Model file for the job. Use its own axes, mm. Face numbers are marked on the shaded views. A direction names the side the tool comes from. Round coordinates to 2 decimals unless told otherwise and drop trailing zeros. Order: outer loops, then holes, each group sorted by start corner. A loop starts at its lowest first (then second) coordinate and runs counter-clockwise, first axis right, second up. Notation, with made-up numbers: M 19.5,0 L 38.5,0 A22 ccw 38.5,21 Z; hole C 23.5,62.25 d11. An arc over 180 degrees is marked long. Return JSON: item names as keys, results as strings. Group by question number.
Item 1: Pull direction X, two halves, no side cores. Call the marked faces 1, 2 and 3: pulls with the +X half, pulls with the -X half, needs draft (parallel to the pull), parting line crosses it, or undercut.
Item 2: Pin check, flat tips, straight feed: pin 1 Ø1.5 at (x, z) = (0, 23) entering from +Y; pin 2 Ø3.5 at (x, z) = (12, 18) entering from -Y; pin 3 Ø0.9 at (x, z) = (-11.5, 16.5) entering from +Y. Stop position of each tip, or through.
Item 3: Slice it at B-B on x = -4.75. Write the cut outline in (y, z).
Item 4: Slice it at A-A on y = 19. Write the cut outline in (x, z).
Item 5: Slice it at D-D on z = 5.5. Write the cut outline in (x, y), then the cut area to 3 significant figures.
Item 6: Slice it at C-C on z = 21.25. Write the cut outline in (x, y), then the cut area to 3 significant figures.
Item 7: Probe line 1 along X through (y, z) = (13.5, 17.75); line 2 along Z through (x, y) = (-10.75, -20); line 3 along Y through (x, z) = (5.75, 10.75). List the from-to ranges inside material, lowest first.
Item 8: Which spindle directions (+Z, -Z, +X, -X, +Y, -Y) get a long thin tool onto all of the face, cutting with end or side? Do the marked faces 4, 5, 6, 7 and 8. Say none if no direction does.
Autodesk Fusion 360 part; units mm, degrees
sketch "Schizzo1" plane through (0, 0, 0) normal (0, 0, 1) x (1, 0, 0)
  line L0 (12.7, -24.75) -> (-12.7, -24.75)
  line L1 (-12.7, -24.75) -> (-12.7, 24.75)
  line L2 (12.7, 24.75) -> (12.7, -24.75)
  line L3 (12.7, -24.75) -> (-12.7, 24.75) construction
  line L4 (-12.7, -24.75) -> (12.7, 24.75) construction
  line L5 (9.7, -18.25) -> (-9.7, -18.25)
  line L6 (9.7, 21.75) -> (9.7, -18.25)
  line L7 (-9.7, -18.25) -> (-9.7, 21.75)
  line L8 (-12.7, 24.75) -> (-9.7, 24.75)
  line L9 (9.7, 24.75) -> (12.7, 24.75)
  line L10 (-9.7, 21.75) -> (-6.7, 21.75)
  line L11 (-6.7, 21.75) -> (-9.7, 24.75)
  line L12 (9.7, 21.75) -> (6.7, 21.75)
  line L13 (6.7, 21.75) -> (9.7, 24.75)
  line L14 (-9.7, -18.25) -> (-12.7, -18.25)
  line L15 (9.7, -18.25) -> (12.7, -18.25)
  line L16 (-9.7, 21.75) -> (-12.7, 21.75)
  line L17 (9.7, 21.75) -> (12.7, 21.75)
  dimension "d15" = 19.4
  dimension "d16" = 3
  dimension "d17" = 3
  dimension "d18" = 6.5
  dimension "d19" = 43
  dimension "d20" = 3
  dimension "d22" = 3
  dimension "d23" = 3
  dimension "d24" = 3
extrude "Estrusione2" add sketch "Schizzo1" along normal blind 25 contours L0 L1 L2 L5 L14 L15 | L2 L6 L15 L17 | L1 L7 L14 L16
extrude "Estrusione3" add sketch "Schizzo1" along normal blind 15 contours L2 L9 L12 L13 L17 | L1 L8 L10 L11 L16
extrude "Estrusione4" cut sketch "Schizzo1" along normal blind 5 from surface at 15 contours L0 L1 L2 L5 L14 L15
chamfer "Smusso1" distance 5 angle 45 2 edges at (11.2, 21.75, 25) (-11.2, 21.75, 25)
sketch "Schizzo2" plane through (0, -24.75, 0) normal (0, -1, 0) x (1, 0, 0)
  line L0 (12.7, 15) -> (-12.7, 15)
  line L1 (-12.7, 15) -> (-12.7, 0)
  line L2 (-12.7, 0) -> (12.7, 0)
  line L3 (12.7, 0) -> (12.7, 15)
  line L4 (0, 15) -> (0, 0) construction
  circle A0 centre (0, 9.5) radius 2.5
  line L5 (-2, 11) -> (2, 11)
  line L6 (-2, 8) -> (2, 8)
  line L7 (-2.5, 9.5) -> (2.5, 9.5) construction
  dimension "d33" = 5
  dimension "d34" = 3
  dimension "d35" = 3
extrude "Estrusione5" cut sketch "Schizzo2" against normal blind 5 contours A0 L5 L6
equation "d17 = d16"
equation "d20 = spessore"
equation "spessore = 3 mm"
equation "d22 = spessore"
equation "d23 = spessore"
equation "d24 = spessore"
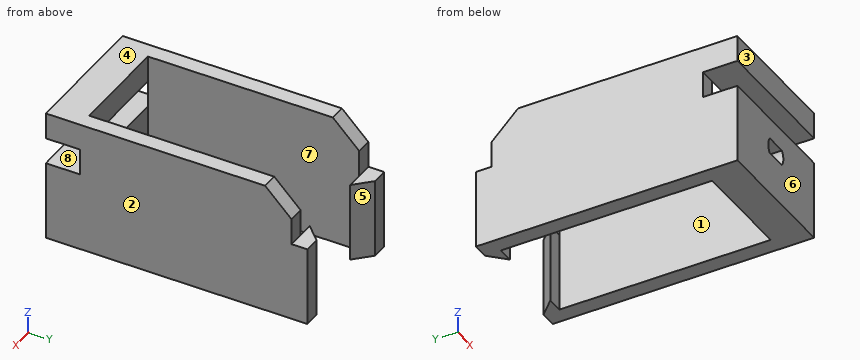
Output values:
{
 "1": {"face 1": "undercut", "face 2": "pulls with the +X half", "face 3": "needs draft"},
 "2": {"pin 1": "y = -18.25", "pin 2": "y = -18.25", "pin 3": "y = 21.75"},
 "3": {"outline": "M -24.75,0 L -18.25,0 L -18.25,15 L -24.75,15 Z; M -24.75,20 L -18.25,20 L -18.25,25 L -24.75,25 Z"},
 "4": {"outline": "M -12.7,0 L -9.7,0 L -9.7,22.75 L -12.7,22.75 Z; M 9.7,0 L 12.7,0 L 12.7,22.75 L 9.7,22.75 Z"},
 "5": {"outline": "M -12.7,-24.75 L 12.7,-24.75 L 12.7,24.75 L 9.7,24.75 L 6.7,21.75 L 9.7,21.75 L 9.7,-18.25 L -9.7,-18.25 L -9.7,21.75 L -6.7,21.75 L -9.7,24.75 L -12.7,24.75 Z", "area": "432 mm²"},
 "6": {"outline": "M -12.7,-24.75 L 12.7,-24.75 L 12.7,20.5 L 9.7,20.5 L 9.7,-18.25 L -9.7,-18.25 L -9.7,20.5 L -12.7,20.5 Z", "area": "398 mm²"},
 "7": {"line 1": "-12.7 to -9.7, 9.7 to 12.7", "line 2": "0 to 15, 20 to 25", "line 3": "-24.75 to -18.25"},
 "8": {"face 4": "+Z, +X, -X, +Y, -Y", "face 5": "+Z, -Z, +Y", "face 6": "+Z, -Z, +X, -X, -Y", "face 7": "+Z, -Z", "face 8": "+X, -X, -Y"}
}
